Check sheet for the modelled part. Datum: model origin and axes. Units: mm. Coordinates: 2 decimals unless noted, no trailing zeros. Loops run counter-clockwise (first coordinate to the right, second up) from the corner with the lowest first, then second, coordinate; pieces in that order, holes last. Notation, with made-up numbers: (-10.75, 57.25) -> (44.25, 57.25) arc R23 cw to (44.25, 71.25) -> close; hole circle Ø6 at (65.25, 7). An arc over 180 degrees is marked (long way). Use one line per item in the form item = value.
from build123d import *


with BuildPart() as part:
    # Sweep1: sweep along a path in Sketch6
    with BuildLine(Plane.XY) as sweep1_path:
        Line((-194.933333333, 26.876190476), (-194.933333333, -83.123809524))
        Line((-194.933333333, -83.123809524), (147.066666667, -83.123809524))
        Line((147.066666667, -83.123809524), (147.066666667, 26.876190476))
        Line((147.066666667, 26.876190476), (-194.933333333, 26.876190476))
    # Sketch7 → Sweep1 (sweep)
    with BuildSketch(Plane(origin=(0, 0, 0), x_dir=(0, 0, -1), z_dir=(1, 0, 0))):
        with BuildLine():
            Line((2.727993364, 26.945293334), (2.497196154, 27.154925683))
            ThreePointArc((2.497196154, 27.154925683), (-0.045784316, 26.049902517), (-2.557836818, 27.223537083))
            Line((-2.557836818, 27.223537083), (-2.798892732, 27.025668774))
            ThreePointArc((-2.798892732, 27.025668774), (-0.053588552, 25.738191345), (2.727993364, 26.945293334))
        make_face()
    sweep(path=sweep1_path.line, transition=Transition.RIGHT)


solid = part.part
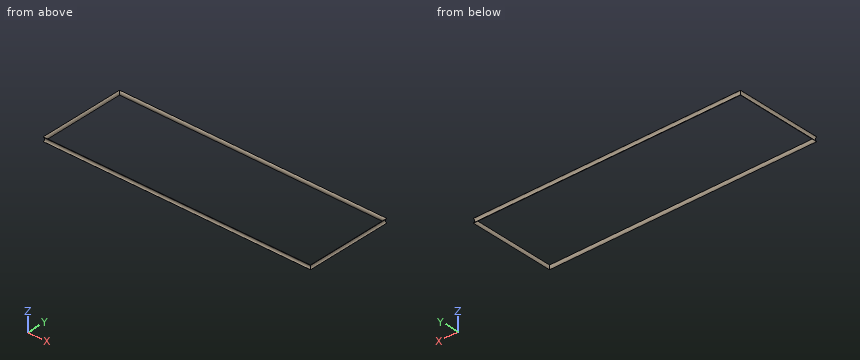
(1) Scan lines: line 1 along Y through (x, z) = (-15, -0.45); line 2 along Y through (x, z) = (-104.5, -0.1); line 3 along X through (y, z) = (-47, 0.6). Record each from-to range of solid material in increasing order.
Established:
line_1 = -82.33 to -82.01, 25.77 to 26.08
line_2 = -82.3 to -81.99, 25.74 to 26.05
line_3 = -194.16 to -193.84, 145.98 to 146.29
(2) Section check C-C, the plane z = 1. Record the boundary of the cut face in (x, y), plus the area to 3 significant figures.
Established:
outline = (-194.26, -82.45) -> (146.39, -82.45) -> (146.39, 26.2) -> (-194.26, 26.2) -> close; hole (-193.93, -82.12) -> (146.07, -82.12) -> (146.07, 25.88) -> (-193.93, 25.88) -> close
area = 292 mm²
(3) Section check B-B, the plane x = 63.5. Record the boundary of the cut face in (y, z).
Established:
outline = (-83.47, 2.56) arc R3.37 cw to (-83.4, -2.5) -> (-83.19, -2.73) arc R3.69 ccw to (-83.27, 2.8) -> close; (26.95, -2.73) -> (27.15, -2.5) arc R3.37 cw to (27.22, 2.56) -> (27.03, 2.8) arc R3.69 ccw to start
(4) Go/stop test with a flat-tipped pin: P1, Ø2, axis at x = -54.5, z = 1.5, coming from the +Y side. Record where the tip stops, or that it passes through.
Established:
P1 = 27.16
(5) Section check A-A, the plane y = 6. Record the boundary of the cut face in (x, z), plus the area to 3 significant figures.
Established:
outline = (-195.28, 2.56) arc R3.37 cw to (-195.21, -2.5) -> (-195, -2.73) arc R3.69 ccw to (-195.08, 2.8) -> close; (147.14, -2.73) -> (147.35, -2.5) arc R3.37 cw to (147.41, 2.56) -> (147.22, 2.8) arc R3.69 ccw to start
area = 3.73 mm²
